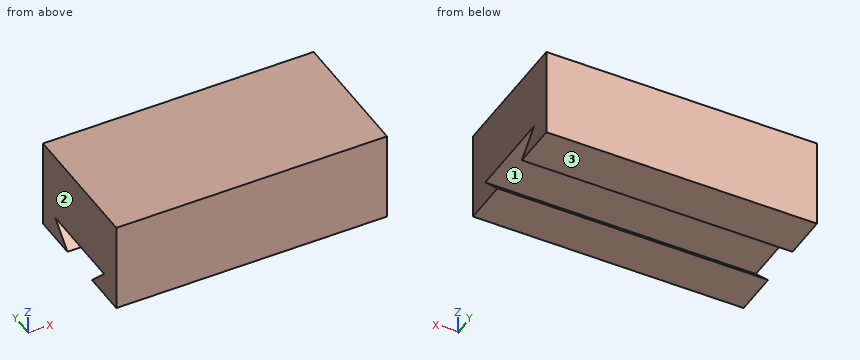
```python
from build123d import *

# Parameters (mm, degrees)
F0_W     = 152.4
F0_H     = 76.2
F1_DEPTH = 50.8
F3_DEPTH = 152.401


with BuildPart() as f1:
    # F0 (on Top) → F1 (new body)
    with BuildSketch(Plane.XY):
        Rectangle(F0_W, F0_H)
    extrude(amount=F1_DEPTH)

    # F2 (on face) → F3 (cut, through all)
    with BuildSketch(Plane.YZ.offset(76.2)):
        Polygon((-25.4, 12.7), (-12.7, 0), (12.7, 0), (25.4, 12.7), align=None)
    extrude(amount=-F3_DEPTH, mode=Mode.SUBTRACT)


solid = f1.part
```
Source: CAD feature listing. Evaluate the final solid. Frame: model axes, mm. Face numbers are marked on the shaded views. Give positions to 0.01 mm unless a question says otherwise; leave off trailing zeros. Loops run counter-clockwise (first coordinate to the right, second up) from the corner with the lowest first, then second, coordinate; pieces in that order, holes last. Notation, with made-up numbers: M 44.5,18.5 L 67.5,18.5 A9 cw 67.5,25.5 Z; hole C 75,34.25 d2. An arc over 180 degrees is marked long. Put each result on its own line as item: value.
Q1. Section C-C (x = 18.5). Return the cut outline in (y, z).
Response values:
outline: M -38.1,0 L -12.7,0 L -25.4,12.7 L 25.4,12.7 L 12.7,0 L 38.1,0 L 38.1,50.8 L -38.1,50.8 Z
Q2. Line query: probe 1 along Z at (x, y) = (64, -19.5); probe 2 along Y at (x, z) = (18, 3.5); probe 3 along Y at (x, z) = (8.5, 6). Output: solid intervals per line, ascending. Write a range as [from, to].
Response values:
probe 1: z = [0, 6.8], [12.7, 50.8]
probe 2: y = [-38.1, -16.2], [16.2, 38.1]
probe 3: y = [-38.1, -18.7], [18.7, 38.1]
Q3. Mould query, pull axis Z, two halves, no side actions, for the marked faces 1, 2 and 3. Classes: released by +Z, released by -Z, zero draft, split by the parting line, or undercut.
Response values:
face 1: undercut
face 2: zero draft
face 3: released by -Z
Q4. Section A-A (z = 6). Return the cut outline in (x, y), and give its area (3 significant figures).
Response values:
outline: M -76.2,-38.1 L 76.2,-38.1 L 76.2,-18.7 L -76.2,-18.7 Z; M -76.2,18.7 L 76.2,18.7 L 76.2,38.1 L -76.2,38.1 Z
area: 5,910 mm²
Q5. Section D-D (y = -9.5). Return the cut outline in (x, z), and give its area (3 significant figures).
Response values:
outline: M -76.2,12.7 L 76.2,12.7 L 76.2,50.8 L -76.2,50.8 Z
area: 5,810 mm²
Q6. Section B-B (y = -23.5). Return the cut outline in (x, z), and give its area (3 significant figures).
Response values:
outline: M -76.2,0 L 76.2,0 L 76.2,10.8 L -76.2,10.8 Z; M -76.2,12.7 L 76.2,12.7 L 76.2,50.8 L -76.2,50.8 Z
area: 7,450 mm²
